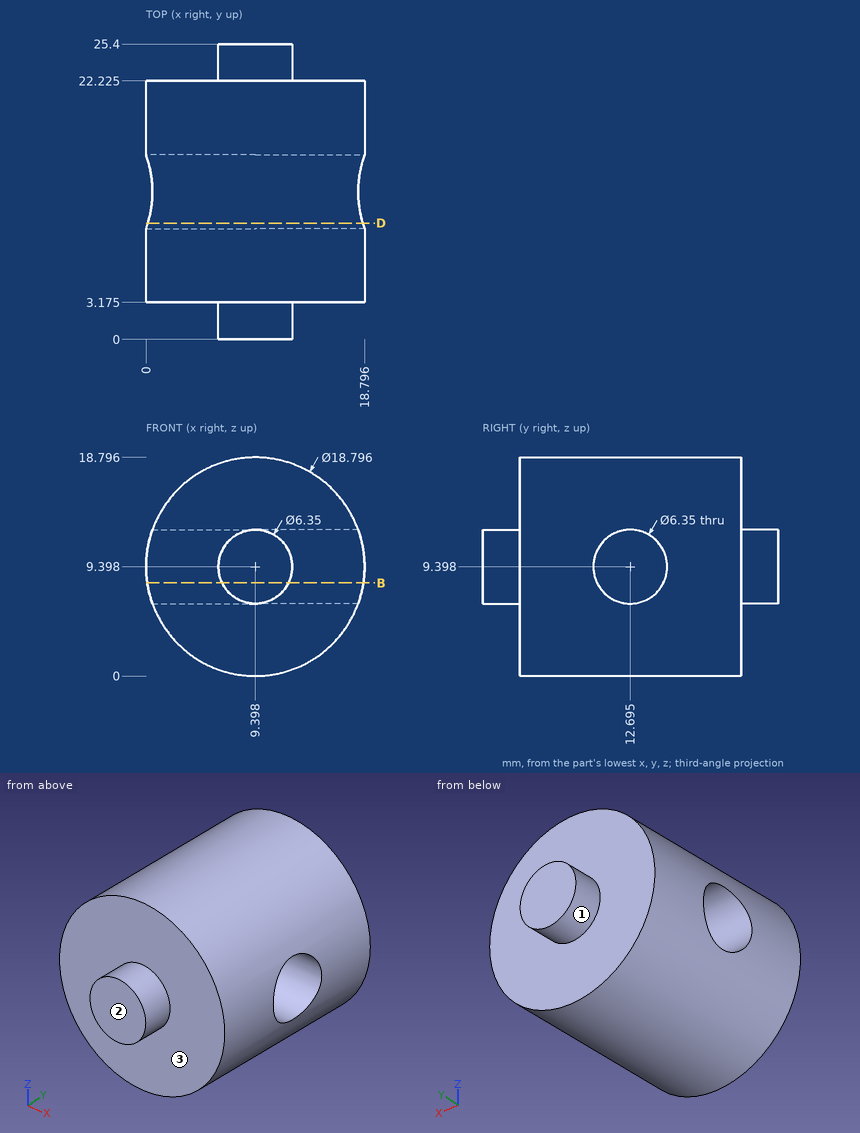
Verification items for this drawing (mm, ordinates from the low corner). A direction names the side the tool comes from. Coordinates: 2 decimals unless noted, no trailing zeros. Loops run counter-clockwise (first coordinate to the right, second up) from the corner with the lowest first, then second, coordinate; pieces in that order, holes last. Notation, with made-up numbers: (84, 65) - (101, 65) arc R30 cw to (101, 94) - close; hole circle Ø11 at (30, 21). An arc over 180 degrees is marked (long way). Answer as a JSON object with one key per item and string values.
(1) Access from +Z, -Z, +X, -X, +Y, -Y to the whole of each face (thin tool, end or side, straight path). Record for the marked faces 1, 2 and 3.
Response:
{"face 1": "+Y", "face 2": "+Z, -Z, +X, -X, -Y", "face 3": "-Y"}
(2) Scan lines: line 1 along Y through (x, z) = (12.75, 1.5) (1 decimal); line 2 along Y through (x, z) = (11.75, 12) (1 decimal); line 3 along Y through (x, z) = (18.25, 9) (1 decimal). Record each from-to range of solid material in increasing order.
Response:
{"line 1": "y = 3.2 to 22.2", "line 2": "y = 3.2 to 10.9, 14.5 to 22.2", "line 3": "y = 3.2 to 9.5, 15.8 to 22.2"}
(3) Go/stop test with flat-tipped pins: pin 1 Ø5 at (x, y) = (15, 15) entering from +Z; pin 2 Ø1 at (y, z) = (8.5, 16) entering from -X; pin 3 Ø10 at (x, z) = (2.5, 16.5) entering from -Y (3 decimals). Record where each tip stops, or that it passes through.
Response:
{"pin 1": "stops at z = 18.27", "pin 2": "stops at x = 2.25", "pin 3": "stops at y = 3.175"}
(4) Cross-section at B-B, the plane z = 8. Record the boundary of the cut face in (x, y) (1 decimal), then the cut area to 3 significant figures.
Response:
{"outline": "(0.1, 3.2) - (6.5, 3.2) - (6.5, 0) - (12.2, 0) - (12.2, 3.2) - (18.7, 3.2) - (18.7, 9.8) - (0.1, 9.8) - close; (0.1, 15.5) - (18.7, 15.5) - (18.7, 22.2) - (12.2, 22.2) - (12.2, 25.4) - (6.5, 25.4) - (6.5, 22.2) - (0.1, 22.2) - close", "area": "284 mm²"}
(5) Cross-section at D-D, the plane y = 10. Record the boundary of the cut face in (x, z) (1 decimal).
Response:
{"outline": "(0.2, 7.7) arc R9.4 ccw to (18.6, 7.7) - close; (0.2, 11.1) - (18.6, 11.1) arc R9.4 ccw to start"}
